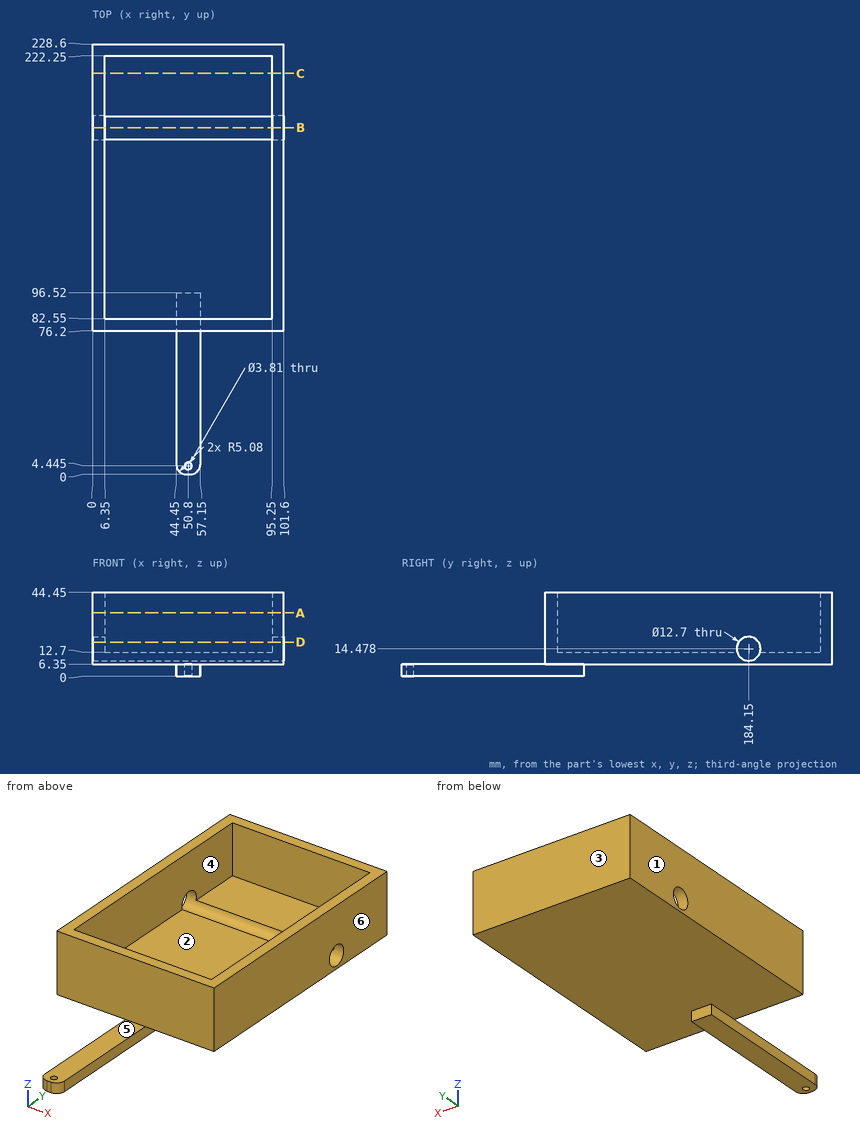
Check sheet for the drawn part. Datum: minimum x, y, z corner. Units: mm. A direction names the side the tool comes from. Round coordinates to 2 decimals unless told otherwise and drop trailing zeros. Write each loop counter-clockwise with the first axis right and the second up, starting at its lowest first coordinate (ties: lowest second). Pieces come first, ordered by that corner, then holes. Notation, with made-up numbers: (20.25, -34.75) - (39.25, -34.75) arc R26 ccw to (39.25, -20.75) - close; hole circle Ø9 at (-16, 79). An arc over 180 degrees is marked (long way). Write each question's results on one line, items separated by ' | '.
(1) Sectioned sample at B-B, the plane y = 184.15. Enter the section's corners in (x, z), plus the area to 3 significant figures.
Computed:
outline: (0, 6.35) - (101.6, 6.35) - (101.6, 8.13) - (0, 8.13) - close; (0, 20.83) - (6.35, 20.83) - (6.35, 44.45) - (0, 44.45) - close; (95.25, 20.83) - (101.6, 20.83) - (101.6, 44.45) - (95.25, 44.45) - close | area: 481 mm^2
(2) Thickness scan on probe 1 along X at (y, z) = (158.5, 32); probe 2 along Y at (x, z) = (67, 40); probe 3 along Y at (x, z) = (50.8, 5). Record the ranges inside material, lowest first. Write a range as from..to.
Computed:
probe 1: x = 0..6.35, 95.25..101.6 | probe 2: y = 76.2..82.55, 222.25..228.6 | probe 3: y = 0..2.54, 6.35..96.52
(3) Draft check along X on the marked faces 1, 2 and 3. Enter one of: pulls with the +X half, pulls with the -X half, needs draft (parallel to the pull), parting line crosses it, or undercut.
Computed:
face 1: pulls with the -X half | face 2: undercut | face 3: needs draft
(4) Set-up check for the marked faces 4, 5 and 6: record each of +Z, -Z, +X, -X, +Y, -Y from which the full face is reachable in a straight line by a thin tool's end or side.
Computed:
face 4: +Z | face 5: +Z, +X, -X, -Y | face 6: +Z, -Z, +X, +Y, -Y
(5) Sectioned sample at D-D, the plane z = 18. Enter the section's corners in (x, y).
Computed:
outline: (0, 76.2) - (101.6, 76.2) - (101.6, 178.87) - (95.25, 178.87) - (95.25, 82.55) - (6.35, 82.55) - (6.35, 178.87) - (0, 178.87) - close; (0, 189.43) - (6.35, 189.43) - (6.35, 222.25) - (95.25, 222.25) - (95.25, 189.43) - (101.6, 189.43) - (101.6, 228.6) - (0, 228.6) - close
(6) Depth check by flat-ended pin: pin 1 Ø1.5 at (x, y) = (46.5, 144.5) entering from +Z; pin 2 Ø7 at (y, z) = (55.5, 2) entering from +X; pin 3 Ø1 at (x, y) = (89, 81) entering from -Z. Enter the tip coordinate at first touch or a pass-through.
Computed:
pin 1: stops at z = 12.7 | pin 2: stops at x = 57.15 | pin 3: stops at z = 6.35
(7) Sectioned sample at A-A, the plane z = 33.5. Enter the section's corners in (x, y), plus the area to 3 significant figures.
Computed:
outline: (0, 76.2) - (101.6, 76.2) - (101.6, 228.6) - (0, 228.6) - close; hole (6.35, 82.55) - (95.25, 82.55) - (95.25, 222.25) - (6.35, 222.25) - close | area: 3,060 mm^2
(8) Sectioned sample at C-C, the plane y = 213. Enter the section's corners in (x, z).
Computed:
outline: (0, 6.35) - (101.6, 6.35) - (101.6, 44.45) - (95.25, 44.45) - (95.25, 12.7) - (6.35, 12.7) - (6.35, 44.45) - (0, 44.45) - close
